Part print with two shaded views. Sizes in mm from the minimum x, y, z corner. A direction names the side the tool comes from. Round coordinates to 2 decimals unless told otherwise and drop trailing zeros. Write each loop counter-clockwise with the first axis right and the second up, starting at its lowest first coordinate (ties: lowest second). Pieces come first, ordered by that corner, then holes. Notation, with made-up numbers: (-39.75, 54.5) -> (-32.75, 54.5) arc R19 cw to (-32.75, 75.5) -> close; hole circle Ø8 at (-32, -32.5). An arc over 180 degrees is marked (long way). Return JSON: item names as keys, results as strings. Group by question number.
(1) Saw through at A-A (y = 5.25). List the corners of the cut face in (x, z), plus the area to 3 significant figures.
(2) Drop flat-ended pins along their axis: pin 1 Ø8 at (x, y) = (15, 9) entering from -Z; pin 2 Ø5 at (x, z) = (15, 8) entering from -Y. Give the stop position or say it passes through.
(3) Saw through at C-C (z = 8). List the corners of the cut face in (x, y), plus the area to 3 significant figures.
(4) Drill centre lines: L1, parallel to Z at x = 1.5, y = 5; L2, parallel to Y at x = 5.5, z = 11. Where is each one in solid material? Low to high. Write a range as from..to.
(5) Tool access for the marked faces 4 and 5: list every direction of +Z, -Z, +X, -X, +Y, -Y with a clear straight run to the whole face (end or side of a thin tool).
(6) Saw through at B-B (x = 6.75). List the corners of the cut face in (y, z).
(7) Mould opens along Z. For the marked faces 1, 2 and 3 say: +Z half, -Z half, draft (parallel to the pull), parting line (faces both ways), or undercut.
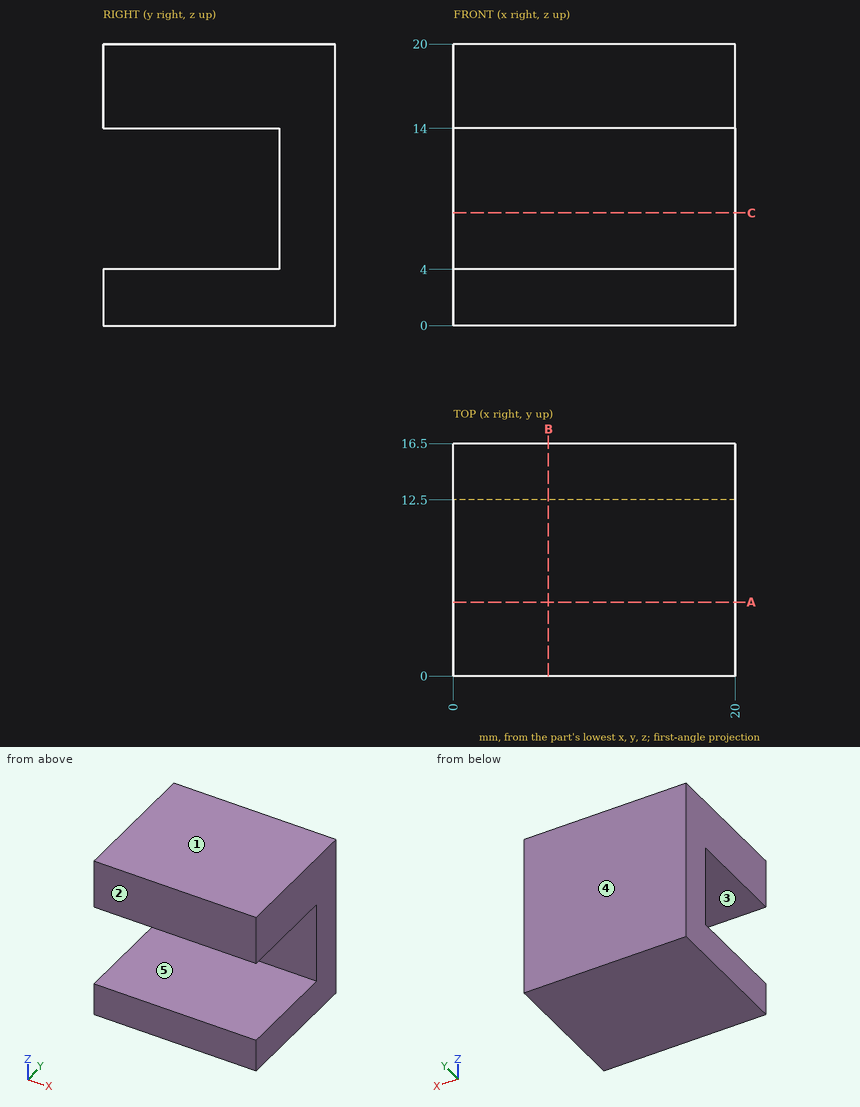
Computed values:
{
 "1": {"outline": "(0, 0) -> (20, 0) -> (20, 4) -> (0, 4) -> close; (0, 14) -> (20, 14) -> (20, 20) -> (0, 20) -> close", "area": "200 mm2"},
 "2": {"pin 1": "z = 0", "pin 2": "y = 12.5"},
 "3": {"outline": "(0, 12.5) -> (20, 12.5) -> (20, 16.5) -> (0, 16.5) -> close", "area": "80.0 mm2"},
 "4": {"L1": "0..4, 14..20", "L2": "12.5..16.5"},
 "5": {"face 4": "+Z, -Z, +X, -X, +Y", "face 5": "+X, -X, -Y"},
 "6": {"outline": "(0, 0) -> (16.5, 0) -> (16.5, 20) -> (0, 20) -> (0, 14) -> (12.5, 14) -> (12.5, 4) -> (0, 4) -> close"},
 "7": {"face 1": "+Z half", "face 2": "draft", "face 3": "undercut"}
}
